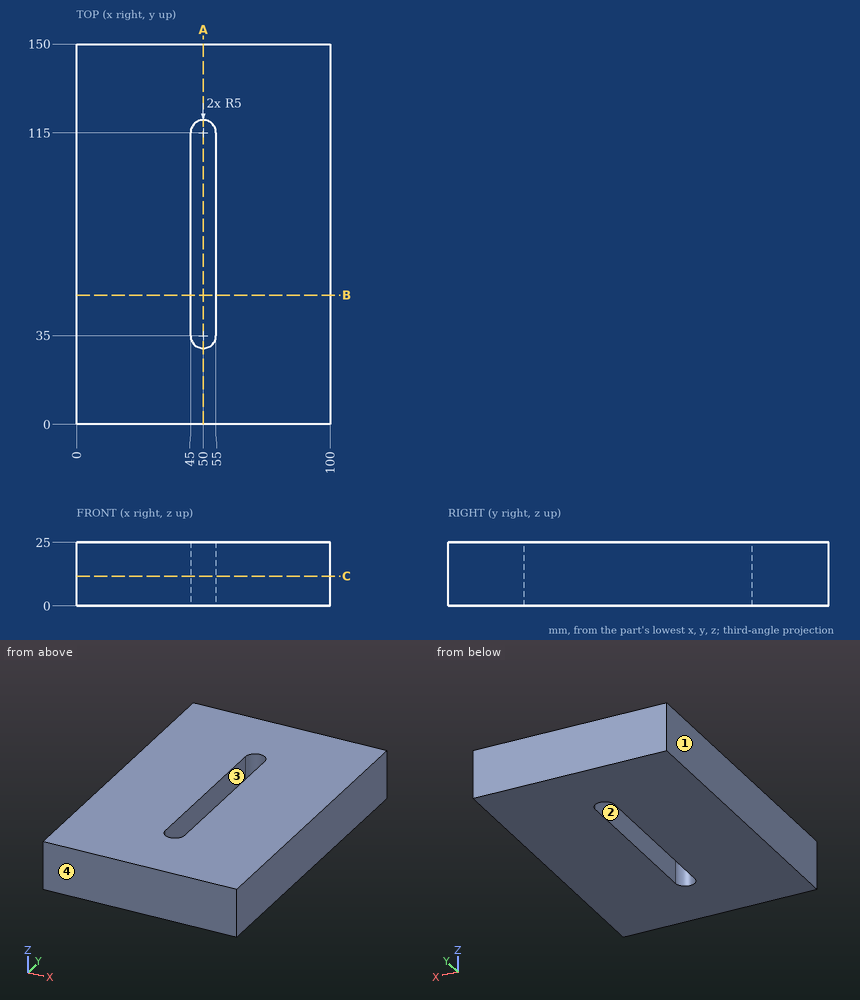
Part print with two shaded views. Sizes in mm from the minimum x, y, z corner. Round coordinates to 2 decimals unless told otherwise and drop trailing zeros. Loops run counter-clockwise (first coordinate to the right, second up) from the corner with the lowest first, then second, coordinate; pieces in that order, holes last.
1. Slice it at A-A (x = 50). Give the cut face in (y, z), and give its area (3 significant figures).
Solutions:
outline: (0, 0) - (30, 0) - (30, 25) - (0, 25) - close; (120, 0) - (150, 0) - (150, 25) - (120, 25) - close
area: 1,500 mm2
2. Slice it at B-B (y = 51). Give the cut face in (x, z).
Solutions:
outline: (0, 0) - (45, 0) - (45, 25) - (0, 25) - close; (55, 0) - (100, 0) - (100, 25) - (55, 25) - close
3. Two-plate mould, pull along X, no slides. Class the marked faces 1, 2, 3 and 4: pulls with the +X half, pulls with the -X half, needs draft (parallel to the pull), parting line crosses it, or undercut.
Solutions:
face 1: pulls with the -X half
face 2: undercut
face 3: undercut
face 4: needs draft
4. Drill centre lines: line 1 along X through (y, z) = (89, 2.25); line 2 along X through (y, z) = (34, 15.5); line 3 along Y through (x, z) = (46.5, 8.75). Where is each one in solid material? Low to high.
Solutions:
line 1: x = 0 to 45, 55 to 100
line 2: x = 0 to 45.1, 54.9 to 100
line 3: y = 0 to 31.43, 118.57 to 150
5. Slice it at C-C (z = 11.75). Give the cut face in (x, y).
Solutions:
outline: (0, 0) - (100, 0) - (100, 150) - (0, 150) - close; hole (45, 35) arc R5 ccw to (55, 35) - (55, 115) arc R5 ccw to (45, 115) - close
